```python
from build123d import *

# Parameters (mm, degrees)
SKETCH1_W           = 31.8
SKETCH1_H           = 15.8
BOSS_EXTRUDE1_DEPTH = 9.6
SKETCH2_W           = 29
SKETCH2_H           = 13.4
CUT_EXTRUDE1_DEPTH  = 8.6
SKETCH3_R           = 2.4
BOSS_EXTRUDE2_DEPTH = 2.8
SKETCH3_3_R         = 1.3
CUT_EXTRUDE2_DEPTH  = 1.7
SKETCH4_R           = 3.25
SKETCH4_R_2         = 2.05
BOSS_EXTRUDE3_DEPTH = 8.6
RIB1_REACH          = 21.951
SKETCH5_WALLS_W     = 1.1
SKETCH5_WALLS_H     = 45.351378422
SKETCH6_W           = 1.2
SKETCH6_H           = 0.2
SKETCH6_W_2         = 0.2
SKETCH6_H_2         = 1.2
BOSS_EXTRUDE4_DEPTH = 8.6


with BuildPart() as part:
    # Sketch1 → Boss-Extrude1 (new body)
    with BuildSketch(Plane(origin=(0, 0, 0), x_dir=(1, 0, 0), z_dir=(0, 1, 0))):
        Rectangle(SKETCH1_W, SKETCH1_H)
    extrude(amount=BOSS_EXTRUDE1_DEPTH)

    # Sketch2 → Cut-Extrude1 (cut)
    with BuildSketch(Plane.XZ):
        Rectangle(SKETCH2_W, SKETCH2_H)
    extrude(amount=-CUT_EXTRUDE1_DEPTH, mode=Mode.SUBTRACT)

    # Sketch3 → Boss-Extrude2 (add)
    with BuildSketch(Plane.XZ.offset(-8.6)):
        with Locations(Location((-12, 4, 0), (0, 0, 270))):
            Circle(SKETCH3_R)
        with Locations(Location((-4, 4, 0), (0, 0, 270))):
            Circle(SKETCH3_R)
        with Locations(Location((4, 4, 0), (0, 0, 270))):
            Circle(SKETCH3_R)
        with Locations(Location((12, 4, 0), (0, 0, 270))):
            Circle(SKETCH3_R)
        with Locations(Location((12, -4, 0), (0, 0, 270))):
            Circle(SKETCH3_R)
        with Locations(Location((4, -4, 0), (0, 0, 270))):
            Circle(SKETCH3_R)
        with Locations(Location((-4, -4, 0), (0, 0, 270))):
            Circle(SKETCH3_R)
        with Locations(Location((-12, -4, 0), (0, 0, 270))):
            Circle(SKETCH3_R)
    extrude(amount=-BOSS_EXTRUDE2_DEPTH)

    # Sketch3<3> → Cut-Extrude2 (cut)
    with BuildSketch(Plane.XZ.offset(-8.6)):
        with Locations(Location((-12, 4, 0), (0, 0, 270))):
            Circle(SKETCH3_3_R)
        with Locations(Location((-4, 4, 0), (0, 0, 270))):
            Circle(SKETCH3_3_R)
        with Locations(Location((4, 4, 0), (0, 0, 270))):
            Circle(SKETCH3_3_R)
        with Locations(Location((12, 4, 0), (0, 0, 270))):
            Circle(SKETCH3_3_R)
        with Locations(Location((12, -4, 0), (0, 0, 270))):
            Circle(SKETCH3_3_R)
        with Locations(Location((4, -4, 0), (0, 0, 270))):
            Circle(SKETCH3_3_R)
        with Locations(Location((-4, -4, 0), (0, 0, 270))):
            Circle(SKETCH3_3_R)
        with Locations(Location((-12, -4, 0), (0, 0, 270))):
            Circle(SKETCH3_3_R)
    extrude(amount=-CUT_EXTRUDE2_DEPTH, mode=Mode.SUBTRACT)

    # Sketch4 → Boss-Extrude3 (add)
    # profile 1 of 3: a face of its own
    with BuildSketch(Plane.XZ.offset(-8.6)):
        with Locations(Location((0, 0, 0), (0, 0, 90))):
            Circle(SKETCH4_R)
        with Locations(Location((0, 0, 0), (0, 0, 90))):
            Circle(SKETCH4_R_2, mode=Mode.SUBTRACT)
    # profile 2 of 3: a face of its own
    with BuildSketch(Plane.XZ.offset(-8.6)):
        with Locations(Location((-8, 0, 0), (0, 0, 90))):
            Circle(SKETCH4_R)
        with Locations(Location((-8, 0, 0), (0, 0, 90))):
            Circle(SKETCH4_R_2, mode=Mode.SUBTRACT)
    # profile 3 of 3: a face of its own
    with BuildSketch(Plane.XZ.offset(-8.6)):
        with Locations(Location((8, 0, 0), (0, 0, 90))):
            Circle(SKETCH4_R)
        with Locations(Location((8, 0, 0), (0, 0, 90))):
            Circle(SKETCH4_R_2, mode=Mode.SUBTRACT)
    extrude(amount=BOSS_EXTRUDE3_DEPTH)

    # Sketch5 walls → Rib1 (add, up to next)
    with BuildSketch(Plane.XZ.offset(-2.3), mode=Mode.PRIVATE) as rib1_sk1:
        with Locations((0, 4.975)):
            Rectangle(SKETCH5_WALLS_W, SKETCH5_WALLS_H)
    rib1_tool1 = extrude(rib1_sk1.sketch, amount=-RIB1_REACH, mode=Mode.PRIVATE) - part.part
    # Sketch5 walls → Rib1 (add, up to next)
    with BuildSketch(Plane.XZ.offset(-2.3), mode=Mode.PRIVATE) as rib1_sk2:
        with Locations((0, -4.975)):
            Rectangle(SKETCH5_WALLS_W, SKETCH5_WALLS_H)
    rib1_tool2 = extrude(rib1_sk2.sketch, amount=-RIB1_REACH, mode=Mode.PRIVATE) - part.part
    add(rib1_tool1.solids().sort_by_distance((0, 2.3, 4.975))[0])
    add(rib1_tool2.solids().sort_by_distance((0, 2.3, -4.975))[0])

    # Sketch6 → Boss-Extrude4 (add)
    with BuildSketch(Plane.XZ):
        with Locations((-12, 6.6)):
            Rectangle(SKETCH6_W, SKETCH6_H)
        with Locations((-4, 6.6)):
            Rectangle(SKETCH6_W, SKETCH6_H)
        with Locations((4, 6.6)):
            Rectangle(SKETCH6_W, SKETCH6_H)
        with Locations((12, 6.6)):
            Rectangle(SKETCH6_W, SKETCH6_H)
        with Locations((12, -6.6)):
            Rectangle(SKETCH6_W, SKETCH6_H)
        with Locations((4, -6.6)):
            Rectangle(SKETCH6_W, SKETCH6_H)
        with Locations((-4, -6.6)):
            Rectangle(SKETCH6_W, SKETCH6_H)
        with Locations((-12, -6.6)):
            Rectangle(SKETCH6_W, SKETCH6_H)
        with Locations((-14.4, -4)):
            Rectangle(SKETCH6_W_2, SKETCH6_H_2)
        with Locations((-14.4, 4)):
            Rectangle(SKETCH6_W_2, SKETCH6_H_2)
        with Locations((14.4, -4)):
            Rectangle(SKETCH6_W_2, SKETCH6_H_2)
        with Locations((14.4, 4)):
            Rectangle(SKETCH6_W_2, SKETCH6_H_2)
    extrude(amount=-BOSS_EXTRUDE4_DEPTH)


solid = part.part
```
For this review, take the finished solid that the model builds, in its own axes (mm). A direction names the side the tool comes from. Round coordinates to 2 decimals unless told otherwise and drop trailing zeros. Write each loop counter-clockwise with the first axis right and the second up, starting at its lowest first coordinate (ties: lowest second). Pieces come first, ordered by that corner, then holes. Notation, with made-up numbers: (32.25, 0) -> (84.25, 0) arc R11 ccw to (84.25, 15) -> close; hole circle Ø5 at (-10.75, 57). An arc over 180 degrees is marked (long way). One line per question, with ' | ' between items. Start each with the question number.
1) Add section B-B (x = 8). Write out the cut boundary in (y, z), and give its area (3 significant figures).
2) Add section A-A (y = 1.25). Count the separate pieces of the cut face and the enclosed holes in it, and give its area (3 significant figures).
3) Machinability: for faces 4 (the cylindrical face through (14.024, 10.487, -5.29)), 5 (the cylindrical face through (-0.98, 4.36, 3.1)), 6 (the flat face through (-12, 11.4, -4)), which of the approach directions +Z, -Z, +X, -X, +Y, -Y give a long, thin tool a straight path to every point of the face, cutting with its end or side? Answer none if there is none.
4) For pin 1 Ø3 at (x, z) = (-12.5, 4.5) entering from -Y; pin 2 Ø1.3 at (x, z) = (-4, 4) entering from -Y, all flat-tipped, find the tip position at first contact; note any pin that passes through.
5) Mouldability with a two-part tool opening along Z and no side actions: class faces 1 (the flat face through (9, 0, 2)), 2 (the flat face through (-4, 4, -6.5)), 3 (the flat face through (0, 5, -7.9)) as +Z half, -Z half, draft (parallel to the pull), parting line (faces both ways), or undercut.
6) Wall thickness on line 1 along X through (y, z) = (9.15, 4); line 2 along X through (y, z) = (7, -3.5); line 3 along X through (y, z) = (7, 6.25): over which ranges is each line inside the solid? List them lowest first.
Reported:
1) outline: (0, -7.9) -> (9.6, -7.9) -> (9.6, 7.9) -> (0, 7.9) -> (0, 6.7) -> (8.6, 6.7) -> (8.6, 3.25) -> (0, 3.25) -> (0, 2.05) -> (8.6, 2.05) -> (8.6, -2.05) -> (0, -2.05) -> (0, -3.25) -> (8.6, -3.25) -> (8.6, -6.7) -> (0, -6.7) -> close | area: 57.1 mm²
2) separate pieces: 4 | enclosed holes: 4 | area: 177 mm²
3) face 4: +Y | face 5: -Y | face 6: +Z, -Z, +X, -X, +Y
4) pin 1: stops at y = 8.6 | pin 2: stops at y = 10.3
5) face 1: draft | face 2: undercut | face 3: -Z half
6) line 1: x = -15.9 to -13.3, -10.7 to -5.3, -2.7 to 2.7, 5.3 to 10.7, 13.3 to 15.9 | line 2: x = -15.9 to -14.3, -0.55 to 0.55, 14.3 to 15.9 | line 3: x = -15.9 to -14.5, -0.55 to 0.55, 14.5 to 15.9
